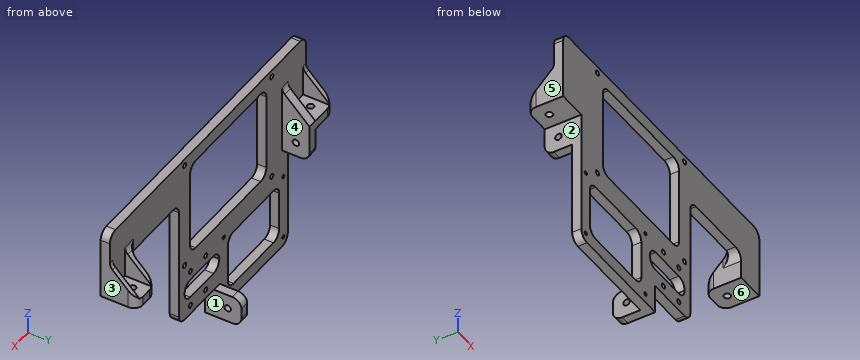
```python
from build123d import *

# Parameters (mm, degrees)
SKETCH2_W            = 217.17
SKETCH2_H            = 49.022
BOSS_EXTRUDE1_DEPTH  = 6.35
SKETCH3_W            = 20.066
SKETCH3_H            = 6.35
BOSS_EXTRUDE2_DEPTH  = 25.4
SKETCH5_W            = 120.65
SKETCH5_H            = 73.406
BOSS_EXTRUDE3_DEPTH  = 6.35
SKETCH6_W            = 6.35
SKETCH6_H            = 26.416
BOSS_EXTRUDE4_DEPTH  = 19.05
SKETCH7_R            = 2.286
CUT_EXTRUDE1_DEPTH   = 134.507689146
SKETCH8_R            = 2.286
CUT_EXTRUDE2_DEPTH   = 222.54657683
SKETCH9_W            = 56.388
SKETCH9_H            = 19.05
CUT_EXTRUDE3_DEPTH   = 148.44946122
SKETCH11_W           = 81.788
SKETCH11_H           = 20.066
BOSS_EXTRUDE5_DEPTH  = 6.35
SKETCH12_W           = 6.35
SKETCH12_H           = 20.066
BOSS_EXTRUDE6_DEPTH  = 25.4
SKETCH16_R           = 1.25
SKETCH16_R_2         = 1.75
SKETCH16_W           = 56.889130435
SKETCH16_H           = 39.65
SKETCH16_W_2         = 84.455
SKETCH16_H_2         = 66.675
SKETCH16_W_3         = 38.360869565
SKETCH16_H_3         = 13.3
CUT_EXTRUDE6_DEPTH   = 162.473195961
BOSS_EXTRUDE8_DEPTH  = 3.175
BOSS_EXTRUDE9_DEPTH  = 3.175
BOSS_EXTRUDE10_DEPTH = 3.175
BOSS_EXTRUDE11_DEPTH = 6.35
FILLET1_R            = 6.35
SKETCH21_R           = 2.286
CUT_EXTRUDE7_DEPTH   = 172.370253676
FILLET2_R            = 6.35


# Some blends are built 0.0001 mm under size
with BuildPart() as part:
    # Sketch2 → Boss-Extrude1 (new body)
    with BuildSketch(Plane(origin=(0, 0, 0), x_dir=(1, 0, 0), z_dir=(0, 1, 0))):
        Rectangle(SKETCH2_W, SKETCH2_H)
    extrude(amount=BOSS_EXTRUDE1_DEPTH)

    # Sketch3 → Boss-Extrude2 (add)
    with BuildSketch(Plane.XZ):
        with Locations((98.552, -21.336)):
            Rectangle(SKETCH3_W, SKETCH3_H)
        with Locations((-98.552, -21.336)):
            Rectangle(SKETCH3_W, SKETCH3_H)
    extrude(amount=-BOSS_EXTRUDE2_DEPTH)

    # Sketch5 → Boss-Extrude3 (add)
    with BuildSketch(Plane(origin=(0, 6.35, 0), x_dir=(1, 0, 0), z_dir=(0, 1, 0))):
        with Locations((-28.194, 61.214)):
            Rectangle(SKETCH5_W, SKETCH5_H)
    extrude(amount=-BOSS_EXTRUDE3_DEPTH)

    # Sketch6 → Boss-Extrude4 (add)
    with BuildSketch(Plane(origin=(0, 6.35, 0), x_dir=(1, 0, 0), z_dir=(0, 1, 0))):
        with Locations((-85.344, 31.369)):
            Rectangle(SKETCH6_W, SKETCH6_H)
    extrude(amount=BOSS_EXTRUDE4_DEPTH)

    # Sketch7 → Cut-Extrude1 (cut, through all)
    with BuildSketch(Plane(origin=(0, 0, -24.511), x_dir=(-1, 0, 0), z_dir=(0, 0, -1))):
        with Locations((-98.552, 15.875)):
            Circle(SKETCH7_R)
        with Locations((98.552, 15.875)):
            Circle(SKETCH7_R)
    extrude(amount=-CUT_EXTRUDE1_DEPTH, mode=Mode.SUBTRACT)

    # Sketch8 → Cut-Extrude2 (cut, through all)
    with BuildSketch(Plane.ZY.offset(88.519)):
        with Locations((-34.544, 15.875)):
            Circle(SKETCH8_R)
    extrude(amount=-CUT_EXTRUDE2_DEPTH, mode=Mode.SUBTRACT)

    # Sketch9 → Cut-Extrude3 (cut, through all)
    with BuildSketch(Plane(origin=(0, 6.35, 0), x_dir=(1, 0, 0), z_dir=(0, 1, 0))):
        with Locations((60.325, 14.986)):
            Rectangle(SKETCH9_W, SKETCH9_H)
    extrude(amount=-CUT_EXTRUDE3_DEPTH, mode=Mode.SUBTRACT)

    # Sketch11 → Boss-Extrude5 (add)
    with BuildSketch(Plane(origin=(0, 6.35, 0), x_dir=(1, 0, 0), z_dir=(0, 1, 0))):
        with Locations((-47.625, 107.95)):
            Rectangle(SKETCH11_W, SKETCH11_H)
    extrude(amount=-BOSS_EXTRUDE5_DEPTH)

    # Sketch12 → Boss-Extrude6 (add)
    with BuildSketch(Plane.XZ):
        with Locations((-9.906, -107.95)):
            Rectangle(SKETCH12_W, SKETCH12_H)
    extrude(amount=-BOSS_EXTRUDE6_DEPTH)

    # Sketch16 → Cut-Extrude6 (cut, through all)
    with BuildSketch(Plane(origin=(0, 6.35, 0), x_dir=(1, 0, 0), z_dir=(0, 1, 0))):
        with Locations(Location((-17.549434783, 111.633, 0), (0, 0, 270))):
            Circle(SKETCH16_R)
        with Locations(Location((-17.549434783, 65.633, 0), (0, 0, 270))):
            Circle(SKETCH16_R)
        with Locations(Location((-83.549434783, 65.633, 0), (0, 0, 270))):
            Circle(SKETCH16_R)
        with Locations(Location((-83.549434783, 111.633, 0), (0, 0, 270))):
            Circle(SKETCH16_R)
        with Locations(Location((-70.739, 56.4515, 0), (0, 0, 270))):
            Circle(SKETCH16_R_2)
        with Locations(Location((-70.739, -19.7485, 0), (0, 0, 270))):
            Circle(SKETCH16_R_2)
        with Locations(Location((25.781, -19.7485, 0), (0, 0, 270))):
            Circle(SKETCH16_R_2)
        with Locations(Location((25.781, 56.4515, 0), (0, 0, 270))):
            Circle(SKETCH16_R_2)
        with Locations(Location((19.431, 91.567, 0), (0, 0, 270))):
            Circle(SKETCH16_R_2)
        with Locations(Location((19.431, 65.567, 0), (0, 0, 270))):
            Circle(SKETCH16_R_2)
        with Locations(Location((2.431, 65.567, 0), (0, 0, 270))):
            Circle(SKETCH16_R_2)
        with Locations(Location((2.431, 91.567, 0), (0, 0, 270))):
            Circle(SKETCH16_R_2)
        with Locations((-50.549434783, 88.633)):
            Rectangle(SKETCH16_W, SKETCH16_H)
        with Locations((-22.479, 18.3515)):
            Rectangle(SKETCH16_W_2, SKETCH16_H_2)
        with Locations((6.600565218, 78.567)):
            Rectangle(SKETCH16_W_3, SKETCH16_H_3)
    extrude(amount=-CUT_EXTRUDE6_DEPTH, mode=Mode.SUBTRACT)

    # Sketch17 → Boss-Extrude8 (add)
    with BuildSketch(Plane.ZY.offset(108.585)):
        Polygon((-18.161, 25.4), (-18.161, 6.35), (0.889, 6.35), align=None)
    extrude(amount=-BOSS_EXTRUDE8_DEPTH)

    # Sketch18 → Boss-Extrude9 (add)
    with BuildSketch(Plane(origin=(108.585, 0, 0), x_dir=(0, 0, -1), z_dir=(1, 0, 0))):
        Polygon((18.161, 25.4), (-0.889, 6.35), (18.161, 6.35), align=None)
    extrude(amount=-BOSS_EXTRUDE9_DEPTH)

    # Sketch19 → Boss-Extrude10 (add)
    with BuildSketch(Plane.ZY.offset(-88.519)):
        Polygon((-18.161, 25.4), (-18.161, 6.35), (0.889, 6.35), align=None)
    extrude(amount=-BOSS_EXTRUDE10_DEPTH)

    # Sketch20 → Boss-Extrude11 (add)
    with BuildSketch(Plane(origin=(-82.169, 0, 0), x_dir=(0, 0, -1), z_dir=(1, 0, 0))):
        Polygon((18.161, 25.4), (-0.889, 6.35), (18.161, 6.35), align=None)
    extrude(amount=-BOSS_EXTRUDE11_DEPTH)

    # Fillet1
    fillet1_edges = [part.edges().sort_by_distance(p)[0] for p in [
        (88.519, 3.175, -5.461),
        (32.131, 3.175, -5.461),
        (-88.519, 3.175, -117.983),
        (-22.104869565, 3.175, -108.458),
        (-22.104869565, 3.175, -68.808),
        (-78.994, 3.175, -68.808),
        (-78.994, 3.175, -108.458),
        (25.781, 3.175, -85.217),
        (25.781, 3.175, -71.917),
        (-12.579869565, 3.175, -71.917),
        (-12.579869565, 3.175, -85.217),
        (19.7485, 3.175, -51.689),
        (19.7485, 3.175, 14.986),
        (-64.7065, 3.175, 14.986),
        (-64.7065, 3.175, -51.689),
        (32.131, 3.175, -97.917),
        (108.585, 3.175, 24.511),
        (-108.585, 3.175, 24.511),
    ]]
    fillet(fillet1_edges, radius=FILLET1_R)

    # Sketch21 → Cut-Extrude7 (cut, through all)
    with BuildSketch(Plane.ZY.offset(13.081)):
        with Locations((-107.95, 15.875)):
            Circle(SKETCH21_R)
    extrude(amount=-CUT_EXTRUDE7_DEPTH, mode=Mode.SUBTRACT)

    # Fillet2
    fillet2_edges = [part.edges().sort_by_distance(p)[0] for p in [
        (88.519, 6.35, -5.461),
        (106.9975, 6.35, 0.889),
        (90.1065, 6.35, 0.889),
        (-85.344, 6.35, 0.889),
        (-106.9975, 6.35, 0.889),
    ]]
    fillet(fillet2_edges, radius=FILLET2_R - 0.0001)  # a hair under: the kernel refuses the full size
    # the kernel refuses this fillet: 6.35 mm, written as the material it takes off along each edge
    with BuildSketch(Plane(origin=(108.585, 25.4, -2.286), x_dir=(0, -1, 0), z_dir=(0, 0, -1)), Plane(origin=(-66.294, 25.4, -44.577), x_dir=(0, -1, 0), z_dir=(-1, 0, 0))) as fillet2_2_piece_1:
        with BuildLine():
            CenterArc((FILLET2_R, FILLET2_R), FILLET2_R, 180, 90)
            Line((0, FILLET2_R), (-FILLET2_R * 0.02, FILLET2_R))
            Line((-FILLET2_R * 0.02, FILLET2_R), (-FILLET2_R * 0.02, -FILLET2_R * 0.02))
            Line((-FILLET2_R * 0.02, -FILLET2_R * 0.02), (FILLET2_R, -FILLET2_R * 0.02))
            Line((FILLET2_R, -FILLET2_R * 0.02), (FILLET2_R, 0))
        make_face()
    extrude(amount=38.1, mode=Mode.SUBTRACT)
    with BuildSketch(Plane(origin=(88.519, 25.4, -40.386), x_dir=(1, 0, 0), z_dir=(0, 0, 1)), Plane(origin=(-28.956, 25.4, -117.983), x_dir=(0, -1, 0), z_dir=(1, 0, 0)), Plane(origin=(-108.585, 25.4, -2.286), x_dir=(0, -1, 0), z_dir=(0, 0, -1)), Plane(origin=(9.144, 25.4, -97.917), x_dir=(0, -1, 0), z_dir=(-1, 0, 0))) as fillet2_2_piece_2:
        with BuildLine():
            CenterArc((FILLET2_R, -FILLET2_R), FILLET2_R, 90, 90)
            Line((0, -FILLET2_R), (-FILLET2_R * 0.02, -FILLET2_R))
            Line((-FILLET2_R * 0.02, -FILLET2_R), (-FILLET2_R * 0.02, FILLET2_R * 0.02))
            Line((-FILLET2_R * 0.02, FILLET2_R * 0.02), (FILLET2_R, FILLET2_R * 0.02))
            Line((FILLET2_R, FILLET2_R * 0.02), (FILLET2_R, 0))
        make_face()
    extrude(amount=38.1, mode=Mode.SUBTRACT)


solid = part.part
```
Verification items for the finished model (mm, model axes). Face numbers are marked on the shaded views. A direction names the side the tool comes from. Round coordinates to 2 decimals unless told otherwise and drop trailing zeros. Loops run counter-clockwise (first coordinate to the right, second up) from the corner with the lowest first, then second, coordinate; pieces in that order, holes last. Notation, with made-up numbers: (17, -19) -> (26, -19) arc R14 ccw to (26, 6) -> close; hole circle Ø2 at (-34, -4). An arc over 180 degrees is marked (long way). Answer as a JSON object with one key per item and string values.
Q1. Section check B-B (x = -45). Record the boundary of the cut face in (y, z), then the cut area to 3 significant figures.
Data:
{"outline": "(0, -117.98) -> (6.35, -117.98) -> (6.35, -108.46) -> (0, -108.46) -> close; (0, -68.81) -> (6.35, -68.81) -> (6.35, -51.69) -> (0, -51.69) -> close; (0, 14.99) -> (6.35, 14.99) -> (6.35, 24.51) -> (0, 24.51) -> close", "area": "230 mm2"}
Q2. Access from +Z, -Z, +X, -X, +Y, -Y to the whole of each face (thin tool, end or side, straight path). Record for the marked faces 1, 2 and 3.
Data:
{"face 1": "-Z, +X, +Y, -Y", "face 2": "-Z, -X, +Y, -Y", "face 3": "+Z, -Z, +X, +Y, -Y"}
Q3. Scan lines: line 1 (Y direction, x = -9.25, z = -107.95); line 2 (Z direction, x = 82.5, y = 4); line 3 (X direction, y = 7.75, z = -100). Record each from-to range of solid material in increasing order. Write a range as from..to.
Data:
{"line 1": "y = 0..13.59, 18.16..25.4", "line 2": "z = -5.47..24.51", "line 3": "x = -13.08..-6.73"}
Q4. Draft check along X on the marked faces 4, 5 and 6. Enter one of: pulls with the +X half, pulls with the -X half, needs draft (parallel to the pull), parting line crosses it, or undercut.
Data:
{"face 4": "undercut", "face 5": "pulls with the -X half", "face 6": "needs draft"}
Q5. Section check D-D (y = 3.25). State how many separate pieces and enclosed holes the cut face has, then the cut area to 3 significant figures.
Data:
{"separate pieces": "1", "enclosed holes": "15", "area": "11,700 mm2"}
Q6. Go/stop test with flat-tipped pins: P1, Ø10, axis at x = 103.5, y = 17.5, coming from the -Z side; P2, Ø1, axis at x = -81, z = -12.5, coming from the +Y side; P3, Ø10, axis at y = 16, z = -47.5, coming from the -X side; P4, Ø1.5, axis at x = -83.55, z = -111.63, coming from the -Y side. Record where each tip stops, or that it passes through.
Data:
{"P1": "stops at z = -24.51", "P2": "stops at y = 6.35", "P3": "stops at x = -88.52", "P4": "passes through"}
Q7. Section check A-A (z = -30). Record the boundary of the cut face in (x, y), then the cut area to 3 significant figures.
Data:
{"outline": "(-88.52, 0) -> (-64.71, 0) -> (-64.71, 6.35) -> (-82.17, 6.35) -> (-82.17, 25.4) -> (-88.52, 25.4) -> close; (19.75, 0) -> (32.13, 0) -> (32.13, 6.35) -> (19.75, 6.35) -> close", "area": "351 mm2"}
